Autodesk Inventor part; units mm, degrees
ref_plane "Work Plane1" through (0, 0, 1.6) normal (0, 0, 1) x (1, 0, 0)
ref_plane "Work Plane2" through (15, 0, 0) normal (1, 0, 0) x (0, 1, 0)
ref_plane "XZ Plane" through (0, 0, 0) normal (0, 1, 0) x (-1, 0, 0)
sketch "Sketch2" plane through (0, 0, 0) normal (0, 1, 0) x (-1, 0, 0)
  line L0 (0, 0) -> (-5, 0)
  line L1 (-5, 0) -> (-10, 1.6)
  line L2 (-10, 1.6) -> (-15, 1.6)
  dimension "d0" = 1.6
  dimension "d1" = 5
  dimension "d2" = 5
  dimension "d3" = 5
sketch "Sketch3" plane through (0, 0, 0) normal (1, 0, 0) x (0, 1, 0)
  circle A0 centre (0, 0) radius 0.9
  dimension "d4" = 1.8
sweep "Sweep1" [suppressed]
ref_plane "Work Plane1" through (0, 0, 1.6) normal (0, 0, 1) x (1, 0, 0)
sketch "Sketch4" plane through (0, 0, 1.6) normal (0, 0, 1) x (1, 0, 0)
  line L0 (25, -15) -> (25, -66.3933)
  line L1 (0, 0) -> (10, 0)
  arc A0 (25, -15) -> (10, 0) centre (10, -15) ccw
  dimension "d33" = 15
  dimension "d34" = 25
  dimension "d35" = 51.3933
ref_plane "Work Plane2" through (15, 0, 0) normal (1, 0, 0) x (0, 1, 0)
sketch "Sketch5" plane through (15, 0, 0) normal (1, 0, 0) x (0, 1, 0)
  circle A0 centre (0, 1.6) radius 0.9
  point P0 (0, 0)
  dimension "d16" = 1.6
  dimension "d17" = 1.8
sweep "Sweep2" [suppressed]
sketch "Sketch7" plane through (0, 0, 0) normal (1, 0, 0) x (0, 1, 0)
  circle A0 centre (0, 0) radius 0.9
  circle A1 centre (0, 0) radius 1.2065
  dimension "d21" = 2.413
extrude "true_tip" add sketch "Sketch7" against normal blind 1
sketch "Sketch8" plane through (-1, 0, 0) normal (-1, 0, 0) x (0, 0, 1)
  circle A0 centre (0, 0) radius 0.9
  circle A1 centre (0, 0) radius 1.2065
  circle A2 centre (0, 0) radius 1
  dimension "d24" = 2
extrude "shoulder_tip" add sketch "Sketch8" along normal blind 2.032 contours A2
sketch "Sketch9" plane through (-3.032, 0, 0) normal (-1, 0, 0) x (0, 0, 1)
  circle A0 centre (0, 0) radius 0.9
  circle A1 centre (0, 0) radius 1
  circle A2 centre (0, 0) radius 1.905
  dimension "d27" = 3.81
extrude "thick" add sketch "Sketch9" along normal blind 8.382 contours A1 | A2
sketch "Sketch10" plane through (-11.414, 0, 0) normal (-1, 0, 0) x (0, 0, 1)
  circle A0 centre (0, 0) radius 0.9
  circle A1 centre (0, 0) radius 1.905
  circle A2 centre (0, 0) radius 1.3462
  dimension "d30" = 2.6924
extrude "thin" add sketch "Sketch10" along normal blind 17.78 contours A2
sketch "Sketch11" plane through (-3.032, 0, 0) normal (1, 0, 0) x (0, 0, -1)
  circle A0 centre (0, 0) radius 1
  line L0 (-1.75, 1.74) -> (1.75, 1.74)
  line L1 (1.75, 1.74) -> (1.75, -1.74)
  line L2 (1.75, -1.74) -> (-1.75, -1.74)
  line L3 (-1.75, -1.74) -> (-1.75, 1.74)
  line L4 (0, 0) -> (1.75, 0)
  line L5 (0, 0) -> (0, 1.74)
  dimension "d36" = 3.48
  dimension "d37" = 3.5
extrude "right_angle" add sketch "Sketch11" along normal blind 4
sketch "Sketch12" plane through (-3.032, -1.74, 1.75) normal (0, 0, 1) x (1, 0, 0)
  line L0 (0, 0) -> (4, 3.48) construction
  line L1 (0, 3.48) -> (4, 0) construction
  circle A0 centre (2, 1.74) radius 1.7526
  point P0 (3.032, 1.74)
  dimension "d40" = 3.5052
extrude "Extrusion6" add sketch "Sketch12" along normal blind 2.032
sketch "Sketch13" plane through (-1.032, 0, 3.782) normal (0, 0, 1) x (1, 0, 0)
  circle A0 centre (0, 0) radius 1.7526
  circle A1 centre (0, 0) radius 1.2065
  circle A2 centre (0, 0) radius 0.8748
  point P0 (1.032, 0)
  dimension "d43" = 2.413
extrude "Extrusion7" add sketch "Sketch13" along normal blind 3.048 contours A1
properties part number "mmcx_ra_coax_tip"
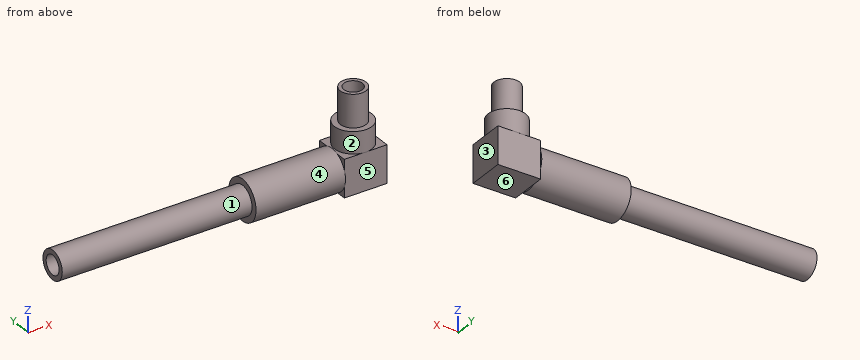
Input: part model. Units: mm. Frame: model coordinates. Face numbers are marked on the shaded views. A direction names the side the tool comes from. Give positions to 0.01 mm unless a question says otherwise; leave off trailing zeros. Order: outer loops, then holes, each group sorted by start corner. A loop starts at its lowest first (then second) coordinate and runs counter-clockwise, first axis right, second up. Notation, with made-up numbers: M 48,63.25 L 96,63.25 A24 ccw 96,78.25 Z; hole C -19,45 d2. An arc over 180 degrees is marked long. Answer as a JSON object with one key per item and string values.
1. Cut plane D-D, the plane z = 5. Output: boundary loops of the cut face in (x, y).
Result sheet:
{"outline": "C -1.03,0 d2.41; hole C -1.03,0 d1.75"}
2. Cut plane B-B, the plane x = -9.5. Output: boundary loops of the cut face in (y, z) (3 decimals), and give its area (3 significant figures).
Result sheet:
{"outline": "C 0,0 d3.81; hole C 0,0 d1.8", "area": "8.86 mm²"}
3. Cut plane A-A, the plane z = 0. Output: boundary loops of the cut face in (x, y) (3 decimals).
Result sheet:
{"outline": "M -29.194,-1.346 L -11.414,-1.346 L -11.414,-1.905 L -3.032,-1.905 L -3.032,-1.74 L 0.968,-1.74 L 0.968,1.74 L -3.032,1.74 L -3.032,1.905 L -11.414,1.905 L -11.414,1.346 L -29.194,1.346 L -29.194,0.9 L -3.032,0.9 L -3.032,-0.9 L -29.194,-0.9 Z"}
4. First-contact query: P1, Ø1, axis at y = 1, z = 4, coming from the +X side; P2, Ø1, axis at x = -1, y = -0.5, coming from the -Z side; P3, Ø2, axis at x = -10.5, z = 1.5, coming from the +Y side; P4, Ø1.4, axis at y = -0.5, z = 0, coming from the -X side. Flat tips, straight axial feed; report the tip coordinate or a pass-through.
Result sheet:
{"P1": "x = 0.63", "P2": "z = -1.75", "P3": "y = 1.84", "P4": "x = -29.19"}
5. Ray query, line 1 (X direction, y = 0.1, z = 5.25); line 2 (Y direction, x = -14.25, z = 0); line 3 (Y direction, x = -11, z = 0) (3 decimals). Return the intervals inside material, ascending. Write a range as [from, to].
Result sheet:
{"line 1": "[-2.23, -1.9], [-0.16, 0.17]", "line 2": "[-1.35, -0.9], [0.9, 1.35]", "line 3": "[-1.905, -0.9], [0.9, 1.905]"}
6. Reachability of the marked faces 1, 2 and 3 from +Z, -Z, +X, -X, +Y, -Y: full face, straight path, thin tool, end or side. Return the list, or none.
Result sheet:
{"face 1": "-X", "face 2": "+Z", "face 3": "+Z, -Z, +X, +Y, -Y"}
7. Pull-direction query (Y, two-part tool) for the marked faces 4, 5 and 6; classes: +Y half, -Y half, draft (parallel to the pull), parting line (faces both ways), or undercut.
Result sheet:
{"face 4": "parting line", "face 5": "-Y half", "face 6": "draft"}
